For this review, take the finished solid that the model builds, in its own axes (mm). Round coordinates to 2 decimals unless told otherwise and drop trailing zeros.
Autodesk Inventor part; units mm, degrees
ref_plane "YZ Plane" through (0, 0, 0) normal (1, 0, 0) x (0, 1, 0)
ref_plane "XZ Plane" through (0, 0, 0) normal (0, 1, 0) x (-1, 0, 0)
ref_plane "XY Plane" through (0, 0, 0) normal (0, 0, 1) x (1, 0, 0)
sketch "Sketch1" plane through (0, 0, 0) normal (0, 1, 0) x (-1, 0, 0)
  line L0 (0, 0) -> (50.8, 0)
  line L1 (50.8, 0) -> (50.8, 76.2)
  line L2 (50.8, 76.2) -> (0, 76.2)
  line L3 (0, 76.2) -> (0, 0)
  circle A0 centre (35.4838, 71.755) radius 2.3813
  circle A1 centre (35.4838, 55.245) radius 2.3813
  circle A2 centre (15.1638, 71.755) radius 2.3813
  circle A3 centre (15.1638, 55.245) radius 2.3813
  line L4 (50.8, 38.1) -> (0, 38.1)
  circle A4 centre (35.4838, 4.445) radius 2.3813
  circle A5 centre (35.4838, 20.955) radius 2.3813
  circle A6 centre (15.1638, 4.445) radius 2.3813
  circle A7 centre (15.1638, 20.955) radius 2.3813
  dimension "d0" = 50.8
  dimension "d1" = 76.2
  dimension "d2" = 4.7625
  dimension "d3" = 15.3162
  dimension "d4" = 4.445
  dimension "d7" = 16.51
  dimension "d10" = 20.32
extrude "Extrusion1" add sketch "Sketch1" along normal blind 3.175
properties part number "Gripper Slider Connecting Plate"
(1) We need section A-A, the plane y = 1.65. State how many separate pieces and enclosed holes the cut face has, and give its area (3 significant figures).
Geometry check:
separate pieces: 1
enclosed holes: 8
area: 3,730 mm2
(2) For line 1 along X through (y, z) = (1, 6.5); line 2 along Z through (x, y) = (-37, 2.85); line 3 along Z through (x, y) = (-13, 2.35), list the stretches that pass through material, from the lowest coordinate up.
Geometry check:
line 1: x = -50.8 to -36.69, -34.28 to -16.37, -13.96 to 0
line 2: z = 0 to 2.61, 6.28 to 19.12, 22.79 to 53.41, 57.08 to 69.92, 73.59 to 76.2
line 3: z = 0 to 3.45, 5.44 to 19.96, 21.95 to 54.25, 56.24 to 70.76, 72.75 to 76.2
(3) For pin 1 Ø8 at (x, z) = (-22.5, 68.5) entering from -Y; pin 2 Ø4.5 at (x, z) = (-15.16, 71.76) entering from +Y, all flat-tipped, find the tip position at first contact; note any pin that passes through.
Geometry check:
pin 1: stops at y = 0
pin 2: passes through
(4) Mouldability with a two-part tool opening along Z and no side actions: class faces 1 (the face through (-25, 2, 0)), 2 (the face through (-37.755, 1.565, 3.73)), 3 (the face through (-25, 0, 39)) as pulls with the +Z half, pulls with the -Z half, needs draft (parallel to the pull), parting line crosses it, or undercut.
Geometry check:
face 1: pulls with the -Z half
face 2: undercut
face 3: needs draft
